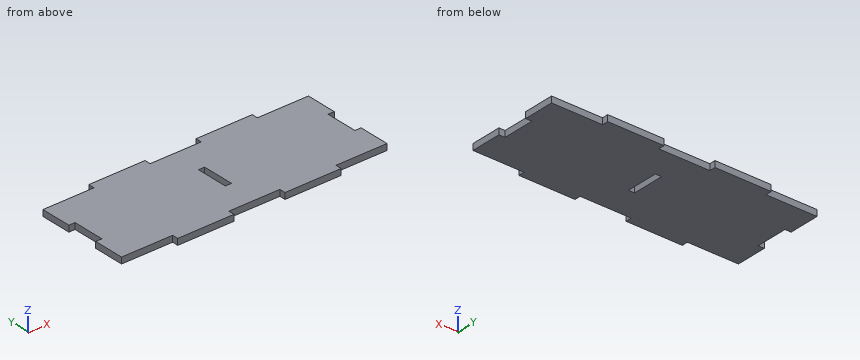
```python
from build123d import *

# Parameters (mm, degrees)
SKETCH_1_W          = 250
SKETCH_1_H          = 88
EXTRUDE_1_DEPTH     = 5.8
CUT_EXTRUDE_1_REACH = 267.099
SKETCH_2_W          = 5.8
SKETCH_2_H          = 30
SKETCH_3_W          = 53
SKETCH_3_H          = 5.8
EXTRUDE_2_DEPTH     = 5.8


with BuildPart() as part:
    # Эскиз1 → Бобышка-Вытянуть1 (new body)
    with BuildSketch(Plane.XY):
        with Locations((125, 44)):
            Rectangle(SKETCH_1_W, SKETCH_1_H)
    extrude(amount=EXTRUDE_1_DEPTH)

    # Эскиз2 → Вырез-Вытянуть1 (cut, up to next)
    with BuildSketch(Plane(origin=(0, 0, 0), x_dir=(-1, 0, 0), z_dir=(0, 0, -1)), mode=Mode.PRIVATE) as cut_extrude_1_sk1:
        with Locations((-247.1, 44)):
            Rectangle(SKETCH_2_W, SKETCH_2_H)
    cut_extrude_1_tool1 = extrude(cut_extrude_1_sk1.sketch, amount=-CUT_EXTRUDE_1_REACH, mode=Mode.PRIVATE) & part.part
    # Эскиз2 → Вырез-Вытянуть1 (cut, up to next)
    with BuildSketch(Plane(origin=(0, 0, 0), x_dir=(-1, 0, 0), z_dir=(0, 0, -1)), mode=Mode.PRIVATE) as cut_extrude_1_sk2:
        with Locations((-125, 44)):
            Rectangle(SKETCH_2_W, SKETCH_2_H)
    cut_extrude_1_tool2 = extrude(cut_extrude_1_sk2.sketch, amount=-CUT_EXTRUDE_1_REACH, mode=Mode.PRIVATE) & part.part
    # Эскиз2 → Вырез-Вытянуть1 (cut, up to next)
    with BuildSketch(Plane(origin=(0, 0, 0), x_dir=(-1, 0, 0), z_dir=(0, 0, -1)), mode=Mode.PRIVATE) as cut_extrude_1_sk3:
        with Locations((-2.9, 44)):
            Rectangle(SKETCH_2_W, SKETCH_2_H)
    cut_extrude_1_tool3 = extrude(cut_extrude_1_sk3.sketch, amount=-CUT_EXTRUDE_1_REACH, mode=Mode.PRIVATE) & part.part
    add(cut_extrude_1_tool1.solids().sort_by_distance((247.1, 44, 0))[0], mode=Mode.SUBTRACT)
    add(cut_extrude_1_tool2.solids().sort_by_distance((125, 44, 0))[0], mode=Mode.SUBTRACT)
    add(cut_extrude_1_tool3.solids().sort_by_distance((2.9, 44, 0))[0], mode=Mode.SUBTRACT)

    # Эскиз3 → Бобышка-Вытянуть2 (add)
    with BuildSketch(Plane.XY.offset(5.8)):
        with Locations((74.5, 90.9)):
            Rectangle(SKETCH_3_W, SKETCH_3_H)
        with Locations((175.5, 90.9)):
            Rectangle(SKETCH_3_W, SKETCH_3_H)
        with Locations((74.5, -2.9)):
            Rectangle(SKETCH_3_W, SKETCH_3_H)
        with Locations((175.5, -2.9)):
            Rectangle(SKETCH_3_W, SKETCH_3_H)
    extrude(amount=-EXTRUDE_2_DEPTH)


solid = part.part
```
Here's how the part is built. I have some questions about the finished solid (model axes, mm). Coordinates: 2 decimals unless noted, no trailing zeros. Order: outer loops, then holes, each group sorted by start corner. A loop starts at its lowest first (then second) coordinate and runs counter-clockwise, first axis right, second up. Notation, with made-up numbers: M 13,-3.5 L 21,-3.5 A29 cw 21,19.5 Z; hole C 48,85.25 d6. An arc over 180 degrees is marked long. Answer as a JSON object with one key per item and string values. Group by question number.
(1) Suppose I cut it at A-A, the plane y = 33. Please give me the cut outline in (x, z).
(2) For pin 1 (3 mm diameter, centred on y = 91, z = 3.5, fed in from -X); pin 2 (1.7 mm diameter, centred on y = 42, z = 3.5, fed in from -X); pin 3 (3 mm diameter, centred on x = 3, z = 2.5, fed in from +Y), each with a flat end and sliding along its axis, tell me the tip position at first contact or that it passes through.
(3) Suppose I cut it at C-C, the plane x = 213. Please give me the cut outline in (y, z), then the cut area to 3 significant figures.
(4) I need wall thicknesses on probe 1 along X at (y, z) = (41.5, 4.25); probe 2 along Y at (x, z) = (219, 4.6). Which ranges of each line are inside material? Lowest first, please.
Values found:
{
 "1": {"outline": "M 5.8,0 L 122.1,0 L 122.1,5.8 L 5.8,5.8 Z; M 127.9,0 L 244.2,0 L 244.2,5.8 L 127.9,5.8 Z"},
 "2": {"pin 1": "stops at x = 48", "pin 2": "stops at x = 5.8", "pin 3": "stops at y = 88"},
 "3": {"outline": "M 0,0 L 88,0 L 88,5.8 L 0,5.8 Z", "area": "510 mm^2"},
 "4": {"probe 1": "x = 5.8 to 122.1, 127.9 to 244.2", "probe 2": "y = 0 to 88"}
}
